from build123d import *

# Parameters (mm, degrees)
MODEL_R         = 2.5999948
MODEL_R_2       = 2.0999958
EXTRUDE_1_DEPTH = 4
EXTRUDE_2_DEPTH = 4
FILLET_1_R      = 10
SKETCH_4_R      = 2.1
EXTRUDE_3_DEPTH = 4
EXTRUDE_4_DEPTH = 4


with BuildPart() as part:
    # Model → Бобышка-Вытянуть1 (new body)
    with BuildSketch(Plane.XY):
        with BuildLine():
            Line((308.392658055, 233.393719024), (308.392658055, 210.464832693))
            ThreePointArc((308.392658055, 210.464832693), (306.92819489, 206.929305859), (303.392668055, 205.464842693))
            Line((303.392668055, 205.464842693), (263.392748055, 205.464842693))
            ThreePointArc((263.392748055, 205.464842693), (259.85722122, 206.929305859), (258.392758055, 210.464832693))
            Line((258.392758055, 210.464832693), (258.392758055, 280.464692693))
            ThreePointArc((258.392758055, 280.464692693), (259.85722122, 284.000219528), (263.392748055, 285.464682693))
            Line((263.392748055, 285.464682693), (273.392728055, 285.464682693))
            ThreePointArc((273.392728055, 285.464682693), (276.92825489, 284.000219528), (278.392718055, 280.464692693))
            Line((278.392718055, 280.464692693), (278.392718055, 270.464712693))
            ThreePointArc((278.392718055, 270.464712693), (279.85718122, 266.929185859), (283.392708055, 265.464722693))
            Line((283.392708055, 265.464722693), (293.392688055, 265.464722693))
            ThreePointArc((293.392688055, 265.464722693), (296.92821489, 264.000259528), (298.392678055, 260.464732693))
            Line((298.392678055, 260.464732693), (298.392678055, 247.535826363))
            ThreePointArc((298.392678055, 247.535826363), (298.773279631, 245.622413028), (299.85714122, 244.000299528))
            Line((299.85714122, 244.000299528), (306.92819489, 236.929245859))
            ThreePointArc((306.92819489, 236.929245859), (308.012056479, 235.307132359), (308.392658055, 233.393719024))
        make_face()
        with Locations((286.392702055, 230.464792693)):
            Circle(MODEL_R, mode=Mode.SUBTRACT)
        with Locations((301.392672055, 215.464822693)):
            Circle(MODEL_R, mode=Mode.SUBTRACT)
        with Locations((268.392738055, 275.464702693)):
            Circle(MODEL_R_2, mode=Mode.SUBTRACT)
        with Locations((268.392738055, 247.464758693)):
            Circle(MODEL_R_2, mode=Mode.SUBTRACT)
        with Locations((288.392698055, 247.464758693)):
            Circle(MODEL_R_2, mode=Mode.SUBTRACT)
    extrude(amount=EXTRUDE_1_DEPTH)

    # Эскиз1 → Бобышка-Вытянуть2 (add)
    with BuildSketch(Plane(origin=(0, 0, 0), x_dir=(-1, 0, 0), z_dir=(0, 0, -1))):
        with BuildLine():
            Line((-308.392658055, 210.464832693), (-308.392658055, 232.615855145))
            Line((-308.392658055, 232.615855145), (-308.392658055, 233.393719024))
            ThreePointArc((-308.392658055, 233.393719024), (-308.012056479, 235.307132359), (-306.92819489, 236.929245859))
            Line((-306.92819489, 236.929245859), (-308.392658055, 236.929245859))
            Line((-308.392658055, 236.929245859), (-320.392658055, 236.929245859))
            Line((-320.392658055, 236.929245859), (-320.392658055, 205.464842693))
            Line((-320.392658055, 205.464842693), (-308.392658055, 205.464842693))
            Line((-308.392658055, 205.464842693), (-303.392668055, 205.464842693))
            ThreePointArc((-303.392668055, 205.464842693), (-306.92819489, 206.929305859), (-308.392658055, 210.464832693))
        make_face()
    extrude(amount=-EXTRUDE_2_DEPTH)

    # Скругление1
    fillet_1_edges = [part.edges().sort_by_distance(p)[0] for p in [
        (306.92819489, 236.929245859, 2),
    ]]
    fillet(fillet_1_edges, radius=FILLET_1_R)

    # Эскиз4 → Бобышка-Вытянуть3 (add)
    with BuildSketch(Plane(origin=(320.392658055, 0, 0), x_dir=(0, 0, -1), z_dir=(1, 0, 0))):
        with BuildLine():
            Line((0, 236.929245859), (-40, 236.929245859))
            ThreePointArc((-40, 236.929245859), (-43.535533906, 235.464779764), (-45, 231.929245859))
            Line((-45, 231.929245859), (-45, 210.464842693))
            ThreePointArc((-45, 210.464842693), (-43.535533906, 206.929308787), (-40, 205.464842693))
            Line((-40, 205.464842693), (0, 205.464842693))
            Line((0, 205.464842693), (0, 236.929245859))
        make_face()
        with Locations(Location((-40, 231.929245859, 0), (0, 0, 90))):
            Circle(SKETCH_4_R, mode=Mode.SUBTRACT)
        with Locations(Location((-40, 210.464842693, 0), (0, 0, 90))):
            Circle(SKETCH_4_R, mode=Mode.SUBTRACT)
        with Locations(Location((-20, 231.929245859, 0), (0, 0, 90))):
            Circle(SKETCH_4_R, mode=Mode.SUBTRACT)
        with Locations(Location((-20, 210.464842693, 0), (0, 0, 90))):
            Circle(SKETCH_4_R, mode=Mode.SUBTRACT)
    extrude(amount=EXTRUDE_3_DEPTH)

    # Эскиз5 → Бобышка-Вытянуть4 (add)
    with BuildSketch(Plane(origin=(0, 236.929245859, 0), x_dir=(1, 0, 0), z_dir=(0, 1, 0))):
        Polygon((320.392658055, -4), (310.392658055, -4), (320.392658055, -14), align=None)
    extrude_4 = extrude(amount=-EXTRUDE_4_DEPTH)

    # Зеркальное отражение1: Бобышка-Вытянуть4 across plane
    add(extrude_4.mirror(Plane.ZX.offset(221.197044276)))


solid = part.part
Input: part model. Units: mm. Frame: model coordinates. A direction names the side the tool comes from. Give positions to 0.01 mm unless a question says otherwise; leave off trailing zeros. Write each loop counter-clockwise with the first axis right and the second up, starting at its lowest first coordinate (ties: lowest second). Pieces come first, ordered by that corner, then holes. Notation, with made-up numbers: M 48.25,32 L 107.25,32 A22 cw 107.25,67 Z; hole C 68,-8 d9. An arc over 180 degrees is marked long. Write item = value, one per line. Start each with the question number.
1) Cut plane B-B on y = 279. Return the cut outline in (x, z), then the cut area to 3 significant figures.
2) Cut plane A-A on z = 20. Return the cut outline in (x, y), then the cut area to 3 significant figures.
3) First-contact query: pin 1 Ø1.5 at (x, y) = (276, 236.5) entering from +Z; pin 2 Ø3.5 at (y, z) = (231.93, 20) entering from -X; pin 3 Ø4.5 at (y, z) = (253.5, 1.5) entering from +X; pin 4 Ø5 at (x, z) = (316.5, 10.5) entering from +Y. Flat tips, straight axial feed; report the tip coordinate or a pass-through.
4) Draft query along Y for faces 1 (the cylindrical face through (296.89, 264.04, 1.97)), 2 (the cylindrical face through (286.84, 248.88, 1.97)), 3 (the flat face through (298.393, 254, 2)). Return one class per face: +Y half, -Y half, draft (parallel to the pull), parting line (faces both ways), or undercut.
5) Cut plane C-C on z = 9. Return the cut outline in (x, y).
6) Cut plane D-D on x = 317. Return the cut outline in (y, z).
7) Material intervals for line 1 along Y through (x, z) = (321, 19); line 2 along Z through (x, y) = (320.5, 210); line 3 along X through (y, z) = (218.5, 16.5), sorted ascending. Write a range as [from, to].
8) Reachability of faces 4 (the flat face through (318, 209.465, 7)), 5 (the flat face through (278.393, 276, 2)), 6 (the flat face through (258.393, 245, 2)) from +Z, -Z, +X, -X, +Y, -Y: full face, straight path, thin tool, end or side. Return the list, or none.
Solved:
q1.outline = M 258.39,0 L 278.39,0 L 278.39,4 L 258.39,4 Z
q1.area = 80.0 mm2
q2.outline = M 320.39,205.46 L 324.39,205.46 L 324.39,208.36 L 320.39,208.36 Z; M 320.39,212.56 L 324.39,212.56 L 324.39,229.83 L 320.39,229.83 Z; M 320.39,234.03 L 324.39,234.03 L 324.39,236.93 L 320.39,236.93 Z
q2.area = 92.3 mm2
q3.pin_1 = 4
q3.pin_2 = through
q3.pin_3 = 298.39
q3.pin_4 = 236.93
q4.face_1 = +Y half
q4.face_2 = undercut
q4.face_3 = draft
q5.outline = M 315.39,205.46 L 324.39,205.46 L 324.39,236.93 L 315.39,236.93 L 315.39,232.93 L 320.39,232.93 L 320.39,209.46 L 315.39,209.46 Z
q6.outline = M 205.46,0 L 236.93,0 L 236.93,10.61 L 232.93,10.61 L 232.93,4 L 209.46,4 L 209.46,10.61 L 205.46,10.61 Z
q7.line_1 = [205.46, 208.62], [212.31, 230.08], [233.78, 236.93]
q7.line_2 = [0, 17.95], [22.05, 37.95], [42.05, 44.98]
q7.line_3 = [320.39, 324.39]
q8.face_4 = +Z, -X
q8.face_5 = +Z, -Z, +X, +Y
q8.face_6 = +Z, -Z, -X, +Y, -Y
